from build123d import *
from build123d import SkipClean  # not in build123d's __all__

# Parameters (mm, degrees)
F0_W      = 140
F0_H      = 85
F0_R      = 8
F1_DEPTH  = 12
F2_W      = 140
F2_H      = 12
F3_DEPTH  = 130
F5_DEPTH  = 18
F7_DEPTH  = 12
F9_DEPTH  = 25
F10_DEPTH = 25
F11_W     = 49
F11_H     = 3
F12_DEPTH = 140.001


# Not quite as in the source:
# - after a boolean that leaves OpenCascade's solid faulty, fix() repairs it
# - a feature of the source that left no trace in its solid (it failed there, or was rolled back) is left out
# - a pattern or mirror of a feature is missing from the dataset's text; its kind, count and spacing are read off the source's solid


with BuildPart() as f1:
    # F0 (on Top) → F1 (new body)
    with BuildSketch(Plane.XY):
        with Locations((70, 42.5)):
            Rectangle(F0_W, F0_H)
        with Locations((35, 30)):
            Circle(F0_R, mode=Mode.SUBTRACT)
        with Locations((105, 30)):
            Circle(F0_R, mode=Mode.SUBTRACT)
    extrude(amount=F1_DEPTH)

    # F2 (on face) → F3 (join)
    with BuildSketch(Plane.XY.offset(12)):
        with Locations((70, 79)):
            Rectangle(F2_W, F2_H)
    extrude(amount=F3_DEPTH)

    # F4 (on face) → F5 (join)
    with BuildSketch(Plane.XZ.offset(-73)):
        with BuildLine():
            ThreePointArc((40, 47), (20, 67), (0, 47))
            ThreePointArc((0, 47), (5.8578643763, 32.8578643763), (20, 27))
            ThreePointArc((20, 27), (34.1421356237, 32.8578643763), (40, 47))
        make_face()
        with BuildLine():
            ThreePointArc((29, 47), (26.3639610307, 40.6360389693), (20, 38))
            ThreePointArc((20, 38), (13.6360389693, 53.3639610307), (29, 47))
        make_face(mode=Mode.SUBTRACT)
    extrude(amount=F5_DEPTH)

    # F6 (on face) → F7 (join)
    with BuildSketch(Plane.XZ.offset(-73)):
        with BuildLine():
            ThreePointArc((117.5, 112), (70.5545635174, 131.4454364826), (90, 84.5))
            ThreePointArc((90, 84.5), (109.4454364826, 92.5545635174), (117.5, 112))
        make_face()
        with BuildLine():
            ThreePointArc((105, 112), (100.6066017178, 101.3933982822), (90, 97))
            ThreePointArc((90, 97), (79.3933982822, 122.6066017178), (105, 112))
        make_face(mode=Mode.SUBTRACT)
    f7 = extrude(amount=F7_DEPTH)

    # F7_copies: F7 across plane
    add(f7.mirror(Plane.ZX.offset(79)), clean=False)

    # F8 (on face) → F9 (cut)
    with BuildSketch(Plane.XZ.offset(-73)):
        with BuildLine():
            Line((62.5, 89.5), (62.5, 112))
            ThreePointArc((62.5, 112), (87.0476647591, 139.3410628291), (116.8660884819, 117.8705442409))
            Line((116.8660884819, 117.8705442409), (140, 12))
            Line((140, 12), (140, 142))
            Line((140, 142), (0, 142))
            Line((0, 142), (0, 47))
            ThreePointArc((0, 47), (5.8578643763, 61.1421356237), (20, 67))
            Line((20, 67), (35.9839461744, 67))
            Line((35.9839461744, 67), (39.2560265726, 67))
            ThreePointArc((39.2560265726, 67), (55.0078493135, 73.9836089388), (62.5, 89.5))
        make_face()
    with SkipClean():  # cleaning this boolean's faces spoils the solid; the shape is the same uncleaned
        extrude(amount=-F9_DEPTH, mode=Mode.SUBTRACT)

    # F10 (cut): faces of the model
    f10_faces = [f1.faces().sort_by_distance(p)[0] for p in [
        (90, 73, 112),
        (20, 73, 47),
    ]]
    extrude(f10_faces, amount=-F10_DEPTH, mode=Mode.SUBTRACT)

    add(f1.part.fix(), mode=Mode.REPLACE)

    # F11 (on face) → F12 (cut, through all)
    with BuildSketch(Plane(origin=(0, 0, 0), x_dir=(0, -1, 0), z_dir=(-1, 0, 0))):
        with Locations((-42.5, 1.5)):
            Rectangle(F11_W, F11_H)
    extrude(amount=-F12_DEPTH, mode=Mode.SUBTRACT)


solid = f1.part
Verification items for the finished model (mm, model axes). A direction names the side the tool comes from. Round coordinates to 2 decimals unless told otherwise and drop trailing zeros. Loops run counter-clockwise (first coordinate to the right, second up) from the corner with the lowest first, then second, coordinate; pieces in that order, holes last. Notation, with made-up numbers: (-21, 46.5) - (-11, 46.5) arc R23 ccw to (-11, 82.5) - close; hole circle Ø9 at (-37.5, -12.75). An arc over 180 degrees is marked (long way). Write item = value, one per line.
Q1. Sectioned sample at A-A on y = 30. Record the boundary of the cut face in (x, z), plus the area to 3 significant figures.
Here are the results:
outline = (0, 3) - (27, 3) - (27, 12) - (0, 12) - close; (43, 3) - (97, 3) - (97, 12) - (43, 12) - close; (113, 3) - (140, 3) - (140, 12) - (113, 12) - close
area = 972 mm^2
Q2. Depth check by flat-ended pin: pin 1 (12 mm diameter, centred on x = 80, z = 60.5, fed in from +Y); pin 2 (2 mm diameter, centred on x = 110, z = 41, fed in from -Y); pin 3 (6 mm diameter, centred on x = 30, y = 77.5, fed in from +Z). Enter the tip coordinate at first touch or a pass-through.
Here are the results:
pin_1 = 85
pin_2 = 73
pin_3 = 67
Q3. Mould release check, pull along Z, two halves, no side actions. Record for faces 5 (the flat face through (69, 76, 0)), 6 (the flat face through (128.27, 78.92, 65.68)), 7 (the flat face through (85, 73, 41)): +Z half, -Z half, draft (parallel to the pull), parting line (faces both ways), or undercut.
Here are the results:
face_5 = -Z half
face_6 = +Z half
face_7 = undercut
Q4. Sectioned sample at B-B on x = 83.5. Record the boundary of the cut face in (y, z).
Here are the results:
outline = (0, 0) - (18, 0) - (18, 3) - (67, 3) - (67, 0) - (85, 0) - (85, 85.28) - (97, 85.28) - (97, 98.48) - (61, 98.48) - (61, 85.28) - (73, 85.28) - (73, 12) - (0, 12) - close; (61, 125.52) - (97, 125.52) - (97, 138.72) - (61, 138.72) - close
Q5. Sectioned sample at C-C on y = 75. Record the boundary of the cut face in (x, z).
Here are the results:
outline = (0, 0) - (140, 0) - (140, 12) - (116.87, 117.87) arc R27.5 ccw to (62.5, 112) - (62.5, 89.5) arc R25 cw to (39.26, 67) - (20, 67) arc R20 ccw to (0, 47) - close; hole circle Ø18 at (20, 47); hole circle Ø30 at (90, 112)
Q6. Material ranges on L1, parallel to X at y = 30, z = 8; L2, parallel to Z at x = 90, y = 65.75; L3, parallel to Z at x = 20, y = 63.25, recorded low to high.
Here are the results:
L1 = 0 to 27, 43 to 97, 113 to 140
L2 = 3 to 12, 84.5 to 97, 127 to 139.5
L3 = 3 to 12, 27 to 38, 56 to 67
Q7. Tool access check on faces 1 (the flat face through (24, 55, 38)), 2 (the flat face through (62.5, 79, 101)), 3 (the flat face through (69, 37, 12)), 4 (the flat face through (69, 43, 3)). Record the directions out of +Z, -Z, +X, -X, +Y, -Y that give a thin tool (end or side, any length) a straight path to the whole face; none if there is none.
Here are the results:
face_1 = +Z, +X, -X, -Y
face_2 = +Z, -X, +Y, -Y
face_3 = +X, -X, -Y
face_4 = -Z, +X, -X
Q8. Sectioned sample at D-D on z = 87.5. Record the boundary of the cut face in (x, y).
Here are the results:
outline = (62.22, 73) - (77.51, 73) - (77.51, 61) - (102.49, 61) - (102.49, 73) - (123.5, 73) - (123.5, 85) - (102.49, 85) - (102.49, 97) - (77.51, 97) - (77.51, 85) - (62.22, 85) - close
